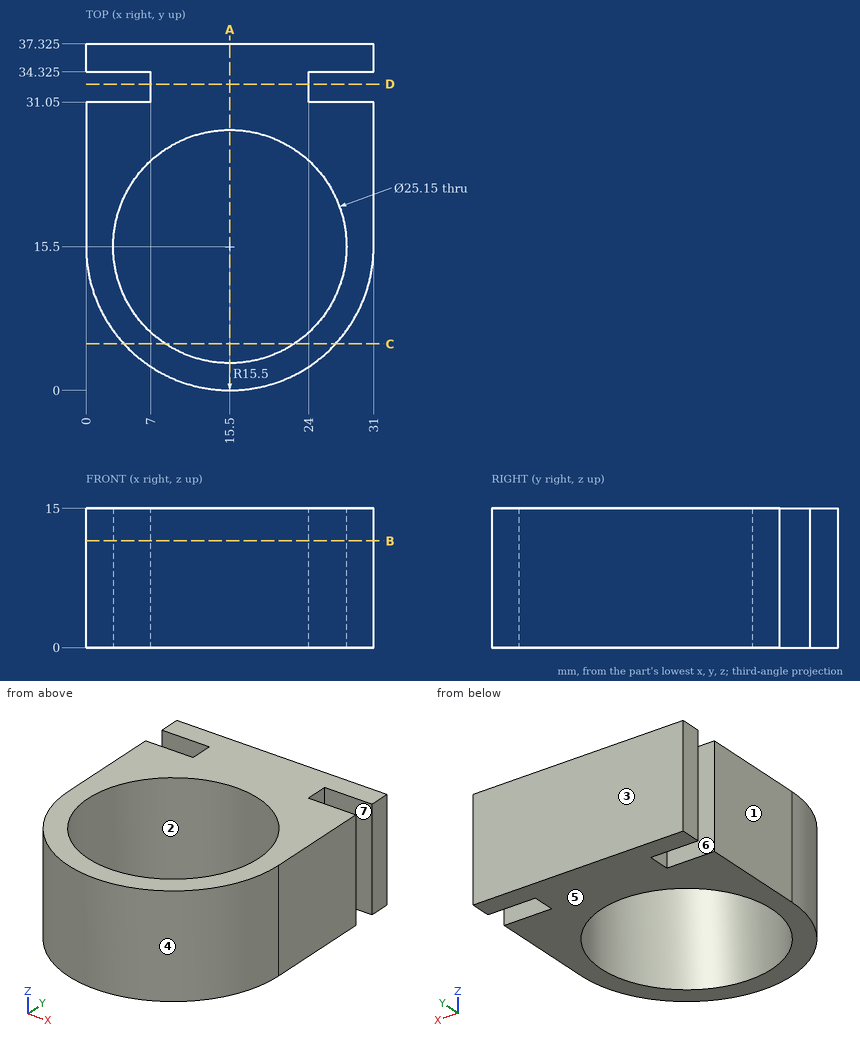
Geometry check sheet. Reference: drawing and pictorial views, mm from the part's lowest x, y, z. A direction names the side the tool comes from. Coordinates: 2 decimals unless noted, no trailing zeros. Write each loop counter-clockwise with the first axis right and the second up, starting at its lowest first coordinate (ties: lowest second). Pieces come first, ordered by that corner, then holes. Notation, with made-up numbers: (-12.75, 89.25) -> (26.25, 89.25) arc R30 cw to (26.25, 128.25) -> close; hole circle Ø3 at (31.5, 36). An arc over 180 degrees is marked (long way). Use a Markdown table: item, result.
1. Release check for a two-part mould opening along X. For the marked faces 1, 2, 3 and 4 record: pulls with the +X half, pulls with the -X half, needs draft (parallel to the pull), parting line crosses it, or undercut.
Reported:
| item | result |
|---|---|
| face 1 | pulls with the -X half |
| face 2 | undercut |
| face 3 | needs draft |
| face 4 | parting line crosses it |
2. Sectioned sample at A-A (x = 15.5). Enter the section's corners in (y, z) (3 decimals).
Reported:
| item | result |
|---|---|
| outline | (0, 0) -> (2.925, 0) -> (2.925, 15) -> (0, 15) -> close; (28.075, 0) -> (37.325, 0) -> (37.325, 15) -> (28.075, 15) -> close |
3. Scan lines: line 1 along Y through (x, z) = (15.5, 4.5) (3 decimals); line 2 along Y through (x, z) = (27, 8.75) (3 decimals); line 3 along X through (y, z) = (15.5, 6.25) (3 decimals). Record each from-to range of solid material in increasing order.
Reported:
| item | result |
|---|---|
| line 1 | y = 0 to 2.925, 28.075 to 37.325 |
| line 2 | y = 5.108 to 10.413, 20.587 to 31.05, 34.325 to 37.325 |
| line 3 | x = 0 to 2.925, 28.075 to 31 |
4. Sectioned sample at C-C (y = 5). Enter the section's corners in (x, z).
Reported:
| item | result |
|---|---|
| outline | (4.1, 0) -> (8.58, 0) -> (8.58, 15) -> (4.1, 15) -> close; (22.42, 0) -> (26.9, 0) -> (26.9, 15) -> (22.42, 15) -> close |
5. Sectioned sample at D-D (y = 33). Enter the section's corners in (x, z).
Reported:
| item | result |
|---|---|
| outline | (7, 0) -> (24, 0) -> (24, 15) -> (7, 15) -> close |
6. Go/stop test with flat-tipped pins: pin 1 Ø5.5 at (x, z) = (28, 5) entering from -Y; pin 2 Ø3.5 at (x, z) = (5, 6) entering from -Y. Record where each tip stops, or that it passes through.
Reported:
| item | result |
|---|---|
| pin 1 | stops at y = 3.45 |
| pin 2 | stops at y = 2.71 |
7. Tool access check on the marked faces 5, 6 and 7. Record the directions out of +Z, -Z, +X, -X, +Y, -Y that give a thin tool (end or side, any length) a straight path to the whole face; none if there is none.
Reported:
| item | result |
|---|---|
| face 5 | -Z, +X, -X, +Y, -Y |
| face 6 | +Z, -Z, -X |
| face 7 | +Z, -Z, +X |
8. Sectioned sample at B-B (z = 11.5). Enter the section's corners in (x, y) (3 decimals).
Reported:
| item | result |
|---|---|
| outline | (0, 15.5) arc R15.5 ccw to (31, 15.5) -> (31, 31.05) -> (24, 31.05) -> (24, 34.325) -> (31, 34.325) -> (31, 37.325) -> (0, 37.325) -> (0, 34.325) -> (7, 34.325) -> (7, 31.05) -> (0, 31.05) -> close; hole circle Ø25.15 at (15.5, 15.5) |
